Here's how the part is built. I have some questions about the finished solid (model axes, mm). Coordinates: 2 decimals unless noted, no trailing zeros. Loops run counter-clockwise (first coordinate to the right, second up) from the corner with the lowest first, then second, coordinate; pieces in that order, holes last. Notation, with made-up numbers: M 51,71.5 L 100,71.5 A7 ccw 100,81.5 Z; hole C -14,-4 d11. An arc over 180 degrees is marked long. Use one line per item in the form item = value. Start each with the question number.
(1) Imagine slicing it at C-C, the plane x = 7. Please give me the cut outline in (y, z).
(2) Imagine slicing it at B-B, the plane y = 25.5. Please give me the cut outline in (x, z), and give its area (3 significant figures).
(3) Will this pin go through, and if not, where does the flat tip stop? P1, Ø0.8, axis at y = 2, z = 1, coming from the -X side.
(4) Imagine slicing it at D-D, the plane z = 0.9. State how many separate pieces and enclosed holes the cut face has, and give its area (3 significant figures).
(5) Imagine slicing it at A-A, the plane y = 65. Please give me the cut outline in (x, z), and give its area (3 significant figures).
(6) Please list where these lines run through material, in increasing order: L1, parallel to X at y = 14, z = 0.45; L2, parallel to X at y = 7.5, z = 0.2; L3, parallel to X at y = -8, z = 0.6.
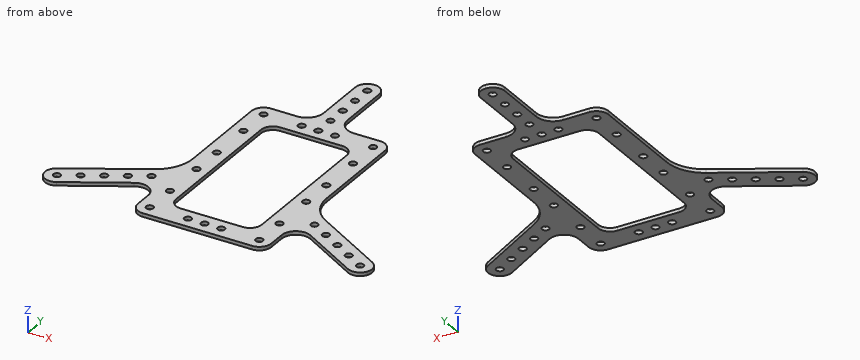
```python
from build123d import *

# Parameters (mm, degrees)
SKETCH_1_R      = 1.5
SKETCH_1_W      = 36
SKETCH_1_H      = 69
EXTRUDE_1_DEPTH = 1.5
FILLET_1_R      = 5
FILLET_2_R      = 6
FILLET_3_R      = 16
FILLET_4_R      = 7
FILLET_5_R      = 5


with BuildPart() as part:
    # 草图1 → 凸台-拉伸1 (new body)
    with BuildSketch(Plane.XY):
        Polygon((28, 44.5), (5, 44.5), (5, 78.5), (-5, 78.5), (-5, 44.5), (-28, 44.5), (-28, -10.392304845), (-70.482994197, -34.919872981), (-65.482994197, -43.580127019), (-28, -21.939310229), (-28, -44.5), (28, -44.5), (28, -21.939310229), (65.482994197, -43.580127019), (70.482994197, -34.919872981), (28, -10.392304845), align=None)
        with Locations((23, -39.5)):
            Circle(SKETCH_1_R, mode=Mode.SUBTRACT)
        with Locations((-23, -39.5)):
            Circle(SKETCH_1_R, mode=Mode.SUBTRACT)
        with Locations((-23, 39.5)):
            Circle(SKETCH_1_R, mode=Mode.SUBTRACT)
        with Locations((23, 39.5)):
            Circle(SKETCH_1_R, mode=Mode.SUBTRACT)
        with Locations((-23, 25.5)):
            Circle(SKETCH_1_R, mode=Mode.SUBTRACT)
        with Locations((23, 25.5)):
            Circle(SKETCH_1_R, mode=Mode.SUBTRACT)
        with Locations((23, -25.5)):
            Circle(SKETCH_1_R, mode=Mode.SUBTRACT)
        with Locations((-23, -25.5)):
            Circle(SKETCH_1_R, mode=Mode.SUBTRACT)
        with Locations((0, 39.5)):
            Circle(SKETCH_1_R, mode=Mode.SUBTRACT)
        with Locations((0, 73.5)):
            Circle(SKETCH_1_R, mode=Mode.SUBTRACT)
        with Locations((-63.652867178, -36.75)):
            Circle(SKETCH_1_R, mode=Mode.SUBTRACT)
        with Locations((-34.208003449, -19.75)):
            Circle(SKETCH_1_R, mode=Mode.SUBTRACT)
        with Locations((63.652867178, -36.75)):
            Circle(SKETCH_1_R, mode=Mode.SUBTRACT)
        with Locations((34.208003449, -19.75)):
            Circle(SKETCH_1_R, mode=Mode.SUBTRACT)
        with Locations((0, -39.5)):
            Circle(SKETCH_1_R, mode=Mode.SUBTRACT)
        with Locations((7, -39.5)):
            Circle(SKETCH_1_R, mode=Mode.SUBTRACT)
        with Locations((-7, -39.5)):
            Circle(SKETCH_1_R, mode=Mode.SUBTRACT)
        with Locations((7, 39.5)):
            Circle(SKETCH_1_R, mode=Mode.SUBTRACT)
        with Locations((-7, 39.5)):
            Circle(SKETCH_1_R, mode=Mode.SUBTRACT)
        with Locations((-23, 7)):
            Circle(SKETCH_1_R, mode=Mode.SUBTRACT)
        with Locations((-23, -7)):
            Circle(SKETCH_1_R, mode=Mode.SUBTRACT)
        with Locations((23, 7)):
            Circle(SKETCH_1_R, mode=Mode.SUBTRACT)
        with Locations((23, -7)):
            Circle(SKETCH_1_R, mode=Mode.SUBTRACT)
        with Locations((0, 65)):
            Circle(SKETCH_1_R, mode=Mode.SUBTRACT)
        with Locations((0, 56.5)):
            Circle(SKETCH_1_R, mode=Mode.SUBTRACT)
        with Locations((0, 48)):
            Circle(SKETCH_1_R, mode=Mode.SUBTRACT)
        with Locations((56.291651246, -32.5)):
            Circle(SKETCH_1_R, mode=Mode.SUBTRACT)
        with Locations((48.930435314, -28.25)):
            Circle(SKETCH_1_R, mode=Mode.SUBTRACT)
        with Locations((41.569219382, -24)):
            Circle(SKETCH_1_R, mode=Mode.SUBTRACT)
        with Locations((-56.291651246, -32.5)):
            Circle(SKETCH_1_R, mode=Mode.SUBTRACT)
        with Locations((-48.930435314, -28.25)):
            Circle(SKETCH_1_R, mode=Mode.SUBTRACT)
        with Locations((-41.569219382, -24)):
            Circle(SKETCH_1_R, mode=Mode.SUBTRACT)
        Rectangle(SKETCH_1_W, SKETCH_1_H, mode=Mode.SUBTRACT)
    extrude(amount=EXTRUDE_1_DEPTH)

    # 圆角1
    fillet_1_edges = [part.edges().sort_by_distance(p)[0] for p in [
        (28, 44.5, 0.75),
        (28, -44.5, 0.75),
        (-28, -44.5, 0.75),
        (-28, 44.5, 0.75),
        (-18, 34.5, 0.75),
        (-18, -34.5, 0.75),
        (18, -34.5, 0.75),
        (18, 34.5, 0.75),
    ]]
    fillet(fillet_1_edges, radius=FILLET_1_R)

    # 圆角2
    fillet_2_edges = [part.edges().sort_by_distance(p)[0] for p in [
        (28, -21.939310229, 0.75),
        (-28, -21.939310229, 0.75),
    ]]
    fillet(fillet_2_edges, radius=FILLET_2_R)

    # 圆角3
    fillet_3_edges = [part.edges().sort_by_distance(p)[0] for p in [
        (28, -10.392304845, 0.75),
        (-28, -10.392304845, 0.75),
    ]]
    fillet(fillet_3_edges, radius=FILLET_3_R)

    # 圆角4
    fillet_4_edges = [part.edges().sort_by_distance(p)[0] for p in [
        (-5, 44.5, 0.75),
        (5, 44.5, 0.75),
    ]]
    fillet(fillet_4_edges, radius=FILLET_4_R)

    # 圆角5
    fillet_5_edges = [part.edges().sort_by_distance(p)[0] for p in [
        (5, 78.5, 0.75),
        (-5, 78.5, 0.75),
        (65.482994197, -43.580127019, 0.75),
        (70.482994197, -34.919872981, 0.75),
        (-65.482994197, -43.580127019, 0.75),
        (-70.482994197, -34.919872981, 0.75),
    ]]
    fillet(fillet_5_edges, radius=FILLET_5_R - 0.0001)  # a hair under: the kernel refuses the full size


solid = part.part
```
Answer:
q1.outline = M -44.5,0 L -41,0 L -41,1.5 L -44.5,1.5 Z; M -38,0 L -34.5,0 L -34.5,1.5 L -38,1.5 Z; M 34.5,0 L 38,0 L 38,1.5 L 34.5,1.5 Z; M 41,0 L 46.6,0 L 46.6,1.5 L 41,1.5 Z
q2.outline = M -28,0 L -24.5,0 L -24.5,1.5 L -28,1.5 Z; M -21.5,0 L -18,0 L -18,1.5 L -21.5,1.5 Z; M 18,0 L 21.5,0 L 21.5,1.5 L 18,1.5 Z; M 24.5,0 L 28,0 L 28,1.5 L 24.5,1.5 Z
q2.area = 21.0 mm²
q3.P1 = -28
q4.separate_pieces = 1
q4.enclosed_holes = 33
q4.area = 3,600 mm²
q5.outline = M -5,0 L -1.5,0 L -1.5,1.5 L -5,1.5 Z; M 1.5,0 L 5,0 L 5,1.5 L 1.5,1.5 Z
q5.area = 10.5 mm²
q6.L1 = -28 to -18, 18 to 28
q6.L2 = -28 to -24.41, -21.59 to -18, 18 to 21.59, 24.41 to 28
q6.L3 = -29.54 to -24.12, -21.88 to -18, 18 to 21.88, 24.12 to 29.54
